from build123d import *

# Parameters (mm, degrees)
SKETCH_W        = 50
SKETCH_H        = 20
SKETCH_R        = 2.1
PAD_DEPTH       = 22
SKETCH001_R     = 11.1
POCKET_DEPTH    = 8
SKETCH002_R     = 5.1
SKETCH002_R_2   = 1.75
POCKET001_DEPTH = 20


with BuildPart() as part:
    # Sketch → Pad (new body)
    with BuildSketch(Plane.XY):
        with Locations((25, 10)):
            Rectangle(SKETCH_W, SKETCH_H)
        with Locations((10, 15)):
            Circle(SKETCH_R, mode=Mode.SUBTRACT)
        with Locations((10, 5)):
            Circle(SKETCH_R, mode=Mode.SUBTRACT)
        with Locations((40, 15)):
            Circle(SKETCH_R, mode=Mode.SUBTRACT)
        with Locations((40, 5)):
            Circle(SKETCH_R, mode=Mode.SUBTRACT)
    extrude(amount=PAD_DEPTH)

    # Sketch001 (on Face3 of Pad) → Pocket (cut)
    with BuildSketch(Plane.XZ):
        with Locations((25, 11)):
            Circle(SKETCH001_R)
    extrude(amount=-POCKET_DEPTH, mode=Mode.SUBTRACT)

    # Sketch002 (on Face1 of Pocket) → Pocket001 (cut)
    with BuildSketch(Plane(origin=(0, 20, 0), x_dir=(-1, 0, 0), z_dir=(0, 1, 0))):
        with Locations((-25, 11)):
            Circle(SKETCH002_R)
        with Locations((-25, 18.95)):
            Circle(SKETCH002_R_2)
        with Locations((-25, 3.05)):
            Circle(SKETCH002_R_2)
        with Locations((-32.95, 11)):
            Circle(SKETCH002_R_2)
        with Locations((-17.05, 11)):
            Circle(SKETCH002_R_2)
    extrude(amount=-POCKET001_DEPTH, mode=Mode.SUBTRACT)


solid = part.part
CAD build for the part. Positions are in the model's coordinates, mm. A direction names the side the tool comes from. Round coordinates to 2 decimals unless told otherwise and drop trailing zeros. Loops run counter-clockwise (first coordinate to the right, second up) from the corner with the lowest first, then second, coordinate; pieces in that order, holes last.
(1) Two-plate mould, pull along Y, no slides. Class faces 3 (the cylindrical face through (26.29, 14.08, 20.13)), 4 (the cylindrical face through (38.452, 16.419, 10.846)), 5 (the flat face through (9, 0, 11)), 6 (the cylindrical face through (37.9, 5.09, 10.85)): +Y half, -Y half, draft (parallel to the pull), parting line (faces both ways), or undercut.
(2) Cut at A-A (z = 11). Give the cut face in (x, y), plus the area to 3 significant figures.
(3) Cut at D-D (y = 1.75). Give the cut face in (x, z), plus the area to 3 significant figures.
(4) Which spindle directions (+Z, -Z, +X, -X, +Y, -Y) get a long thin tool onto all of the face, cutting with end or side? Do faces 1 (the flat face through (50, 10, 11)), 2 (the cylindrical face through (36.1, 3.9, 10.8)). Say none if no direction does.
(5) Wall check: line 1 along Y through (x, z) = (10, 11.25); line 2 along X through (y, z) = (6, 10.5); line 3 along Z through (x, y) = (23.5, 15). Give the ranges that are in metal, low to high.
(6) Cut at B-B (y = 5). Give the cut face in (x, z).
(7) Drop flat-ended pins along their axis: pin 1 (3 mm diameter, centred on x = 17.05, z = 11, fed in from -Y); pin 2 (6.5 mm diameter, centred on x = 10, y = 5, fed in from +Z); pin 3 (4.5 mm diameter, centred on x = 32.95, z = 11, fed in from -Y). Give the stop position or say it passes through.
(8) Cut at C-C (x = 25). Give the cut face in (y, z).
Findings below:
1. face 3: draft
1. face 4: undercut
1. face 5: -Y half
1. face 6: undercut
2. outline: (0, 0) - (13.9, 0) - (13.9, 8) - (15.3, 8) - (15.3, 20) - (0, 20) - close; (18.8, 8) - (19.9, 8) - (19.9, 20) - (18.8, 20) - close; (30.1, 8) - (31.2, 8) - (31.2, 20) - (30.1, 20) - close; (34.7, 8) - (36.1, 8) - (36.1, 0) - (50, 0) - (50, 20) - (34.7, 20) - close; hole circle Ø4.2 at (10, 5); hole circle Ø4.2 at (10, 15); hole circle Ø4.2 at (40, 5); hole circle Ø4.2 at (40, 15)
2. area: 561 mm2
3. outline: (0, 0) - (23.51, 0) arc R11.1 cw to (23.51, 22) - (0, 22) - close; (26.49, 0) - (50, 0) - (50, 22) - (26.49, 22) arc R11.1 cw to start
3. area: 713 mm2
4. face 1: +Z, -Z, +X, +Y, -Y
4. face 2: -Y
5. line 1: y = 0 to 2.9, 7.1 to 12.9, 17.1 to 20
5. line 2: x = 0 to 8.15, 11.85 to 13.91, 36.09 to 38.15, 41.85 to 50
5. line 3: z = 0 to 2.15, 3.95 to 6.13, 15.87 to 18.05, 19.85 to 22
6. outline: (0, 0) - (7.9, 0) - (7.9, 22) - (0, 22) - close; (12.1, 0) - (23.51, 0) arc R11.1 cw to (23.51, 22) - (12.1, 22) - close; (26.49, 0) - (37.9, 0) - (37.9, 22) - (26.49, 22) arc R11.1 cw to start; (42.1, 0) - (50, 0) - (50, 22) - (42.1, 22) - close
7. pin 1: passes through
7. pin 2: stops at z = 22
7. pin 3: stops at y = 8
8. outline: (8, 0) - (20, 0) - (20, 1.3) - (8, 1.3) - close; (8, 4.8) - (20, 4.8) - (20, 5.9) - (8, 5.9) - close; (8, 16.1) - (20, 16.1) - (20, 17.2) - (8, 17.2) - close; (8, 20.7) - (20, 20.7) - (20, 22) - (8, 22) - close
